Verification items for this drawing (mm, ordinates from the low corner). A direction names the side the tool comes from. Give positions to 0.01 mm unless a question says otherwise; leave off trailing zeros. Order: outer loops, then holes, each group sorted by start corner. A loop starts at its lowest first (then second) coordinate and runs counter-clockwise, first axis right, second up. Notation, with made-up numbers: M -6,-24.5 L -2,-24.5 A16 cw -2,-11.5 Z; hole C -18.5,-27.75 d4. An arc over 180 degrees is marked long. Return JSON: item names as keys, results as strings. Group by question number.
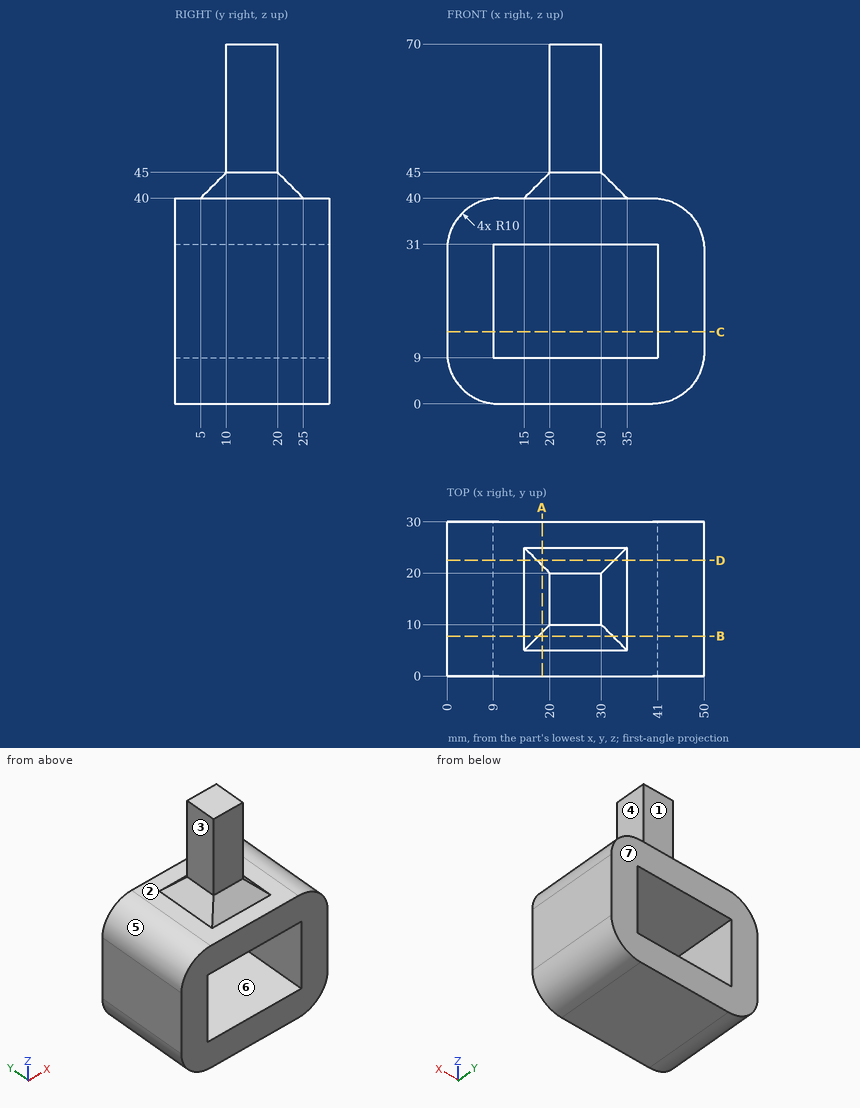
1) Release check for a two-part mould opening along X. For the marked faces 4, 5, 6 and 7 record: released by +X, released by -X, zero draft, split by the parting line, or undercut.
2) Sectioned sample at B-B on y = 7.75. Record the boundary of the cut face in (x, z), then the cut area to 3 significant figures.
3) Tool access check on the marked faces 1, 2 and 3. Record the directions out of +Z, -Z, +X, -X, +Y, -Y that give a thin tool (end or side, any length) a straight path to the whole face; none if there is none.
4) Sectioned sample at D-D on y = 22.5. Record the boundary of the cut face in (x, z), then the cut area to 3 significant figures.
5) Material ranges on line 1 along Z through (x, y) = (18, 26.25); line 2 along X through (y, z) = (12, 12.5); line 3 along Z through (x, y) = (25, 13.5), recorded low to high.
6) Depth check by flat-ended pin: P1, Ø1.5, axis at x = 38.5, y = 26.5, coming from the +Z side; P2, Ø8, axis at y = 17.5, z = 52.5, coming from the +X side; P3, Ø8, axis at x = 25.5, z = 55.5, coming from the +Y side. Enter the tip coordinate at first touch or a pass-through.
7) Sectioned sample at A-A on x = 18.5. Record the boundary of the cut face in (y, z), then the cut area to 3 significant figures.
8) Sectioned sample at C-C on z = 14. Record the boundary of the cut face in (x, y), then the cut area to 3 significant figures.
Reply:
{
 "1": {"face 4": "released by +X", "face 5": "released by -X", "face 6": "undercut", "face 7": "zero draft"},
 "2": {"outline": "M 0,10 A10 ccw 10,0 L 40,0 A10 ccw 50,10 L 50,30 A10 ccw 40,40 L 35,40 L 32.25,42.75 L 17.75,42.75 L 15,40 L 10,40 A10 ccw 0,30 Z; hole M 9,9 L 41,9 L 41,31 L 9,31 Z", "area": "1,260 mm^2"},
 "3": {"face 1": "+Z, +X, -X, +Y", "face 2": "+Z", "face 3": "+Z, -X, +Y, -Y"},
 "4": {"outline": "M 0,10 A10 ccw 10,0 L 40,0 A10 ccw 50,10 L 50,30 A10 ccw 40,40 L 35,40 L 32.5,42.5 L 17.5,42.5 L 15,40 L 10,40 A10 ccw 0,30 Z; hole M 9,9 L 41,9 L 41,31 L 9,31 Z", "area": "1,250 mm^2"},
 "5": {"line 1": "0 to 9, 31 to 40", "line 2": "0 to 9, 41 to 50", "line 3": "0 to 9, 31 to 70"},
 "6": {"P1": "z = 40", "P2": "x = 30", "P3": "y = 20"},
 "7": {"outline": "M 0,0 L 30,0 L 30,9 L 0,9 Z; M 0,31 L 30,31 L 30,40 L 25,40 L 21.5,43.5 L 8.5,43.5 L 5,40 L 0,40 Z", "area": "598 mm^2"},
 "8": {"outline": "M 0,0 L 9,0 L 9,30 L 0,30 Z; M 41,0 L 50,0 L 50,30 L 41,30 Z", "area": "540 mm^2"}
}
